Geometry: final body of the model. Coordinates: model frame, mm. A direction names the side the tool comes from. Give positions to 0.01 mm unless a question says otherwise; leave off trailing zeros. Write each loop counter-clockwise with the first axis right and the second up, starting at its lowest first coordinate (ties: lowest second). Pieces come first, ordered by that corner, then holes. Notation, with made-up numbers: (64, 55.5) -> (77, 55.5) arc R17 cw to (77, 77.5) -> close; hole circle Ø7 at (45.5, 66). An arc over 180 degrees is marked (long way). Answer in a Markdown table with one row per item. Add a question column.
from build123d import *

# Parameters (mm, degrees)
F1_DEPTH = 63.5
F0_W     = 25.4
F0_H     = 19.05
F2_DEPTH = 25.4
F3_DEPTH = 7.9375
F5_R     = 6.35


# Not quite as in the source:
# - a feature names something its author has since deleted; it is built from what else it names


with BuildPart() as f1:
    # F0 (on Front) → F1 (new body, symmetric)
    with BuildSketch(Plane.XZ):
        Polygon((-41.275, 9.525), (-41.275, -9.525), (41.275, -9.525), (41.275, 9.525), (22.225, 9.525), align=None)
    extrude(amount=F1_DEPTH, both=True)

    # F0 (on Front) → F2 (join, symmetric)
    with BuildSketch(Plane.XZ):
        with BuildLine():
            Line((22.225, 9.525), (41.275, 9.525))
            Line((41.275, 9.525), (41.275, 27.0002))
            ThreePointArc((41.275, 27.0002), (45.9246798487, 38.2255201513), (57.15, 42.8752))
            Line((57.15, 42.8752), (60.325, 42.8752))
            Line((60.325, 42.8752), (60.325, 61.9252))
            Line((60.325, 61.9252), (57.15, 61.9252))
            ThreePointArc((57.15, 61.9252), (32.4542956671, 51.6959043329), (22.225, 27.0002))
            Line((22.225, 27.0002), (22.225, 9.525))
        make_face()
        with Locations((73.025, 52.4002)):
            Rectangle(F0_W, F0_H)
    extrude(amount=F2_DEPTH, both=True)

    # F0 (on Front) → F3 (join, symmetric)
    with BuildSketch(Plane.XZ):
        with BuildLine():
            add(Edge.make_bspline(
                [(-41.275, 9.525), (-33.0378338695, 42.7445545793), (5.4129776545, 65.891072154), (57.15, 61.9252)],
                knots=[0, 0, 0, 0, 111.5045361635, 111.5045361635, 111.5045361635, 111.5045361635], degree=3))
            Line((-41.275, 9.525), (22.225, 9.525))
            Line((22.225, 9.525), (22.225, 27.0002))
            ThreePointArc((22.225, 27.0002), (32.4542956671, 51.6959043329), (57.15, 61.9252))
        make_face()
    extrude(amount=F3_DEPTH, both=True)

    # F0 (on Front) → F4 (revolve)
    with BuildSketch(Plane.XZ):
        Polygon((85.725, 66.675), (85.725, 61.9252), (85.725, 42.8752), (85.725, 38.1), (111.125, 38.1), (111.125, 66.675), align=None)
    revolve(axis=Axis((85.725, 0, 52.3875), (0, 0, 1)))

    # F5
    f5_edges = [f1.edges().sort_by_distance(p)[0] for p in [
        (41.275, -63.5, 0),
        (-41.275, -63.5, 0),
        (41.275, 63.5, 0),
        (-41.275, 63.5, 0),
    ]]
    fillet(f5_edges, radius=F5_R)


solid = f1.part
Q1. Section B-B on x = 65.5. Return loops of the section in (y, z) (3 decimals).
Q2. Section C-C on y = -29.5. Return loops of the section in (x, z) (3 decimals), and give its area (3 significant figures).
Q3. Section A-A on z = 2.5. Return loops of the section in (x, y) (3 decimals), and give its area (3 significant figures).
Q4. Pull-direction query (X, two-part tool) for faces 6 (the flat face through (22.225, 17, 18)), 7 (the cylindrical face through (39.464, 61.59, 0.133)), 8 (the flat face through (1, 35, 9.525)), 9 (the flat face through (60, 2, 42.875)); classes: +X half, -X half, draft (parallel to the pull), parting line (faces both ways), or undercut.
Q5. Contact query for flat-ended pins moving along their axis: pin 1 Ø5 at (y, z) = (17, 18.5) entering from -X (3 decimals); pin 2 Ø19 at (y, z) = (-20.5, 18) entering from -X (3 decimals); pin 3 Ø3 at (x, z) = (88, 46) entering from -Y; pin 4 Ø15 at (x, y) = (74.5, 1.5) entering from -Z. Output: stop coordinate, or through.
Q6. Line query: probe 1 along Y at (x, z) = (-25.5, 28); probe 2 along X at (y, z) = (-12, -3) (3 decimals); probe 3 along X at (y, z) = (-9, 21) (3 decimals). Output: solid intervals per line, ascending. Write a range as from..to.
Q7. Access query for faces 1 (the flat face through (46, 25.4, 42)), 2 (the flat face through (-41.275, -1, 0)), 3 (the flat face through (-2, 7.938, 32)), 4 (the flat face through (41.275, -1, 4)), 5 (the cylindrical face through (32.73, -16.79, 51.97)). Directions: +Z, -Z, +X, -X, +Y, -Y. A direction counts if a zero-diameter tool reaches every point of the face in a straight line with its end or side. Return the directions, or none.
Checks:
| question | item | result |
|---|---|---|
| 1 | outline | (-25.4, 42.875) -> (-15.366, 42.875) -> (-15.366, 38.1) -> (15.366, 38.1) -> (15.366, 42.875) -> (25.4, 42.875) -> (25.4, 61.925) -> (15.366, 61.925) -> (15.366, 66.675) -> (-15.366, 66.675) -> (-15.366, 61.925) -> (-25.4, 61.925) -> close |
| 2 | outline | (-41.275, -9.525) -> (41.275, -9.525) -> (41.275, 9.525) -> (-41.275, 9.525) -> close |
| 2 | area | 1,570 mm^2 |
| 3 | outline | (-41.275, -57.15) arc R6.35 ccw to (-34.925, -63.5) -> (34.925, -63.5) arc R6.35 ccw to (41.275, -57.15) -> (41.275, 57.15) arc R6.35 ccw to (34.925, 63.5) -> (-34.925, 63.5) arc R6.35 ccw to (-41.275, 57.15) -> close |
| 3 | area | 10,400 mm^2 |
| 4 | face 6 | -X half |
| 4 | face 7 | +X half |
| 4 | face 8 | draft |
| 4 | face 9 | undercut |
| 5 | pin 1 | x = 22.225 |
| 5 | pin 2 | x = -41.275 |
| 5 | pin 3 | y = -25.39 |
| 5 | pin 4 | z = 38.1 |
| 6 | probe 1 | -7.94..7.94 |
| 6 | probe 2 | -41.275..41.275 |
| 6 | probe 3 | 22.225..41.275 |
| 7 | face 1 | +Z, +X, -X, +Y |
| 7 | face 2 | +Z, -Z, -X, +Y, -Y |
| 7 | face 3 | +Z, -X, +Y |
| 7 | face 4 | -Z, +X, +Y, -Y |
| 7 | face 5 | +Z, -X, -Y |
